from build123d import *

# Parameters (mm, degrees)
F0_R     = 5
F0_R_2   = 2
F1_DEPTH = 8
F3_DEPTH = 3


with BuildPart() as f1:
    # F0 (on Top) → F1 (new body)
    with BuildSketch(Plane.XY):
        with BuildLine():
            ThreePointArc((3.984848, 22.652174), (0, 27), (-3.984848, 22.652174))
            ThreePointArc((-3.984848, 22.652174), (-23, 0), (-3.984848, -22.652174))
            ThreePointArc((-3.984848, -22.652174), (0, -27), (3.984848, -22.652174))
            ThreePointArc((3.984848, -22.652174), (23, 0), (3.984848, 22.652174))
        make_face()
        Circle(F0_R, mode=Mode.SUBTRACT)
        with Locations((8, 0)):
            Circle(F0_R_2, mode=Mode.SUBTRACT)
    extrude(amount=F1_DEPTH)

    # F2 (on face) → F3 (cut)
    with BuildSketch(Plane.XY.offset(8)):
        with BuildLine():
            ThreePointArc((-3.984848, 22.652174), (0, 23), (3.984848, 22.652174))
            ThreePointArc((3.984848, 22.652174), (0, 27), (-3.984848, 22.652174))
        make_face()
        with BuildLine():
            ThreePointArc((-3.984848, -22.652174), (0, -27), (3.984848, -22.652174))
            ThreePointArc((3.984848, -22.652174), (0, -23), (-3.984848, -22.652174))
        make_face()
    extrude(amount=-F3_DEPTH, mode=Mode.SUBTRACT)


solid = f1.part
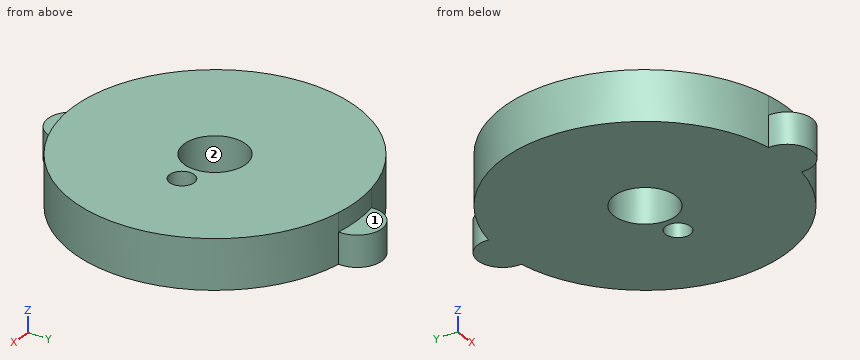
Model file for the job. Use its own axes, mm. Face numbers are marked on the shaded views. Give positions to 0.01 mm unless a question says otherwise; leave off trailing zeros. Order: outer loops, then holes, each group sorted by start corner. A loop starts at its lowest first (then second) coordinate and runs counter-clockwise, first axis right, second up. Notation, with made-up numbers: (7, -25) - (29, -25) arc R25 cw to (29, -13) - close; hole circle Ø7 at (30.5, 69.5). An arc over 180 degrees is marked (long way). Return JSON: item names as keys, results as strings.
1) Probe line 1 (X direction, y = 1, z = 4); line 2 (Y direction, x = 3, z = 7.5); line 3 (X direction, y = 11.5, z = 4.25). List the from-to ranges inside material, lowest first. Write a range as from..to.
Geometry says:
{"line 1": "-22.98..-4.9, 4.9..6.27, 9.73..22.98", "line 2": "-22.8..-4, 4..22.8", "line 3": "-19.92..19.92"}
2) Pull direction Y, two halves, no side cores. Call the marked faces 1 and 2: pulls with the +Y half, pulls with the -Y half, needs draft (parallel to the pull), parting line crosses it, or undercut.
Geometry says:
{"face 1": "needs draft", "face 2": "undercut"}
3) Cut at C-C, the plane z = 0.75. Give the cut face in (x, y), plus the area to 3 significant figures.
Geometry says:
{"outline": "(-3.98, -22.65) arc R4 ccw (long way) to (3.98, -22.65) arc R23 ccw to (3.98, 22.65) arc R4 ccw (long way) to (-3.98, 22.65) arc R23 ccw to start; hole circle Ø10 at (0, 0); hole circle Ø4 at (8, 0)", "area": "1,620 mm²"}
4) Cut at A-A, the plane x = 0. Give the cut face in (y, z), plus the area to 3 significant figures.
Geometry says:
{"outline": "(-27, 0) - (-5, 0) - (-5, 8) - (-23, 8) - (-23, 5) - (-27, 5) - close; (5, 0) - (27, 0) - (27, 5) - (23, 5) - (23, 8) - (5, 8) - close", "area": "328 mm²"}
5) Cut at D-D, the plane x = 8. Give the cut face in (y, z), plus the area to 3 significant figures.
Geometry says:
{"outline": "(-21.56, 0) - (-2, 0) - (-2, 8) - (-21.56, 8) - close; (2, 0) - (21.56, 0) - (21.56, 8) - (2, 8) - close", "area": "313 mm²"}
6) Flat gauge pins, fed straight in: P1, Ø1.3, axis at x = -1, y = 25, coming from the +Z side; P2, Ø1.5, axis at y = -11.5, z = 4.5, coming from the -X side; P3, Ø2, axis at y = -3.5, z = 7, coming from the +X side. Where does each tip first touch, or does it go through?
Geometry says:
{"P1": "z = 5", "P2": "x = -20.33", "P3": "x = 22.86"}
7) Cut at B-B, the plane y = 0. Give the cut face in (x, z).
Geometry says:
{"outline": "(-23, 0) - (-5, 0) - (-5, 8) - (-23, 8) - close; (5, 0) - (6, 0) - (6, 8) - (5, 8) - close; (10, 0) - (23, 0) - (23, 8) - (10, 8) - close"}
